from build123d import *

# Parameters (mm, degrees)
F1_DEPTH = 74
F2_W     = 12
F2_H     = 44
F3_DEPTH = 2
F4_W     = 12
F4_H     = 2
F5_DEPTH = 25
F7_DEPTH = 8


with BuildPart() as f1:
    # F0 (on Right) → F1 (new body)
    with BuildSketch(Plane.YZ):
        with BuildLine():
            ThreePointArc((-26.041336, 5), (-23.041336, 8), (-26.041336, 11))
            Line((-26.041336, 11), (-26.041336, 15))
            ThreePointArc((-26.041336, 15), (-23.920016, 15.87868), (-23.041336, 18))
            Line((-23.041336, 18), (-9.041336, 18))
            ThreePointArc((-9.041336, 18), (-8.162657, 15.87868), (-6.041336, 15))
            Line((-6.041336, 15), (-6.041336, 11))
            ThreePointArc((-6.041336, 11), (-9.041336, 8), (-6.041336, 5))
            Line((-6.041336, 5), (5.958664, 5))
            Line((5.958664, 5), (5.958664, 30))
            Line((5.958664, 30), (-38.041336, 30))
            Line((-38.041336, 30), (-38.041336, 5))
            Line((-38.041336, 5), (-26.041336, 5))
        make_face()
    extrude(amount=F1_DEPTH)

    # F2 (on face) → F3 (cut)
    with BuildSketch(Plane.XY.offset(30)):
        with Locations((68, -16.041336)):
            Rectangle(F2_W, F2_H)
        with Locations((6, -16.041336)):
            Rectangle(F2_W, F2_H)
    extrude(amount=-F3_DEPTH, mode=Mode.SUBTRACT)

    # F4 (on face) → F5 (cut)
    with BuildSketch(Plane.XY.offset(30)):
        with Locations((6, 4.958664)):
            Rectangle(F4_W, F4_H)
        with Locations((6, -37.041336)):
            Rectangle(F4_W, F4_H)
        with Locations((68, -37.041336)):
            Rectangle(F4_W, F4_H)
        with Locations((68, 4.958664)):
            Rectangle(F4_W, F4_H)
    extrude(amount=-F5_DEPTH, mode=Mode.SUBTRACT)

    # F6 (on face) → F7 (cut)
    with BuildSketch(Plane.XY.offset(30)):
        with BuildLine():
            ThreePointArc((21.5, -0.041336), (17.232233, 1.726431), (19, -2.541336))
            ThreePointArc((19, -2.541336), (20.767767, -1.809103), (21.5, -0.041336))
        make_face()
        with BuildLine():
            ThreePointArc((52.5, -0.041336), (53.232233, -1.809103), (55, -2.541336))
            ThreePointArc((55, -2.541336), (56.767767, -1.809103), (57.5, -0.041336))
            ThreePointArc((57.5, -0.041336), (55, 2.458664), (52.5, -0.041336))
        make_face()
        with BuildLine():
            ThreePointArc((55, -29.541336), (53.232233, -30.273569), (52.5, -32.041336))
            ThreePointArc((52.5, -32.041336), (55, -34.541336), (57.5, -32.041336))
            ThreePointArc((57.5, -32.041336), (56.767767, -30.273569), (55, -29.541336))
        make_face()
        with BuildLine():
            ThreePointArc((19, -29.541336), (17.232233, -33.809103), (21.5, -32.041336))
            ThreePointArc((21.5, -32.041336), (20.767767, -30.273569), (19, -29.541336))
        make_face()
    extrude(amount=-F7_DEPTH, mode=Mode.SUBTRACT)


solid = f1.part
For this review, take the finished solid that the model builds, in its own axes (mm). A direction names the side the tool comes from. Round coordinates to 2 decimals unless told otherwise and drop trailing zeros. Write each loop counter-clockwise with the first axis right and the second up, starting at its lowest first coordinate (ties: lowest second). Pieces come first, ordered by that corner, then holes. Notation, with made-up numbers: (61, -13.75) -> (85, -13.75) arc R21 cw to (85, 3.25) -> close; hole circle Ø11 at (42, 59). An arc over 180 degrees is marked (long way). Use CSV: the item, a comma, the result in double quotes.
(1) To check wall thickness, follow L1, parallel to Y at x = 19, z = 24.5; L2, parallel to Y at x = 43.5, z = 13; L3, parallel to Y at x = 11, z = 13.5. State the ranges of each line that lie inside material, in increasing order. Write a range as [from, to].
Computed values:
L1,"[-38.04, -34.54], [-29.54, -2.54], [2.46, 5.96]"
L2,"[-38.04, -26.04], [-6.04, 5.96]"
L3,"[-36.04, -26.04], [-6.04, 3.96]"
(2) Consider section C-C, the plane y = -25. Give the boundary of the cut face in (x, z).
Computed values:
outline,"(0, 5.19) -> (74, 5.19) -> (74, 10.81) -> (0, 10.81) -> close; (0, 15.19) -> (74, 15.19) -> (74, 28) -> (62, 28) -> (62, 30) -> (12, 30) -> (12, 28) -> (0, 28) -> close"
(3) Draft analysis for pull direction Z (two halves, no side actions). For faces 5 (the face through (12, -18, 29)), 6 (the face through (36, -6.041, 13)), 7 (the face through (19, 0, 22)), state which applies: +Z half, -Z half, draft (parallel to the pull), parting line (faces both ways), or undercut.
Computed values:
face 5,"draft"
face 6,"undercut"
face 7,"+Z half"
(4) Consider section A-A, the plane z = 8. Give the boundary of the cut face in (x, y), plus the area to 3 significant figures.
Computed values:
outline,"(0, -36.04) -> (12, -36.04) -> (12, -38.04) -> (62, -38.04) -> (62, -36.04) -> (74, -36.04) -> (74, -23.04) -> (0, -23.04) -> close; (0, -9.04) -> (74, -9.04) -> (74, 3.96) -> (62, 3.96) -> (62, 5.96) -> (12, 5.96) -> (12, 3.96) -> (0, 3.96) -> close"
area,"2,120 mm²"
(5) Clearance check with flat-ended pins moving along their axes: P1, Ø4, axis at x = 64.5, z = 7.5, coming from the -Y side; P2, Ø6, axis at x = 5.5, z = 22, coming from the +Y side; P3, Ø1.5, axis at x = 54, y = 0, coming from the +Z side. State where each tip first meets the part, or that it passes through.
Computed values:
P1,"y = -36.04"
P2,"y = 3.96"
P3,"z = 22"
(6) For faces 1 (the face through (55, 0, 22)), 2 (the face through (36.482, -8.186, 15.902)), 3 (the face through (68, -16, 28)), 4 (the face through (6, -36.041, 17)), list the 3-axis set-ups (+Z, -Z, +X, -X, +Y, -Y) from which the entire face can be reached by the end or side of a thin tool; tool diameter is ignored.
Computed values:
face 1,"+Z"
face 2,"+X, -X"
face 3,"+Z, +X, +Y, -Y"
face 4,"+Z, -Z, -X, -Y"
(7) Consider section D-D, the plane x = 9. Give the boundary of the cut face in (y, z).
Computed values:
outline,"(-36.04, 5) -> (-26.04, 5) arc R3 ccw to (-26.04, 11) -> (-26.04, 15) arc R3 ccw to (-23.04, 18) -> (-9.04, 18) arc R3 ccw to (-6.04, 15) -> (-6.04, 11) arc R3 ccw to (-6.04, 5) -> (3.96, 5) -> (3.96, 28) -> (-36.04, 28) -> close"
(8) Consider section B-B, the plane z = 24. Give the boundary of the cut face in (x, y).
Computed values:
outline,"(0, -36.04) -> (12, -36.04) -> (12, -38.04) -> (62, -38.04) -> (62, -36.04) -> (74, -36.04) -> (74, 3.96) -> (62, 3.96) -> (62, 5.96) -> (12, 5.96) -> (12, 3.96) -> (0, 3.96) -> close; hole circle Ø5 at (19, -32.04); hole circle Ø5 at (19, -0.04); hole circle Ø5 at (55, -32.04); hole circle Ø5 at (55, -0.04)"
